The drawing under review shows one solid part. Ordinate dimensions are in mm from its lowest x, y, z. A direction names the side the tool comes from. Coordinates: 2 decimals unless noted, no trailing zeros. Order: outer loops, then holes, each group sorted by start corner. A loop starts at its lowest first (then second) coordinate and runs counter-clockwise, first axis right, second up. Notation, with made-up numbers: (51.5, 24) -> (107.5, 24) arc R22 cw to (107.5, 56) -> close; hole circle Ø8 at (88, -28.75). An arc over 180 degrees is marked (long way). Put each result on its own line as item: value.
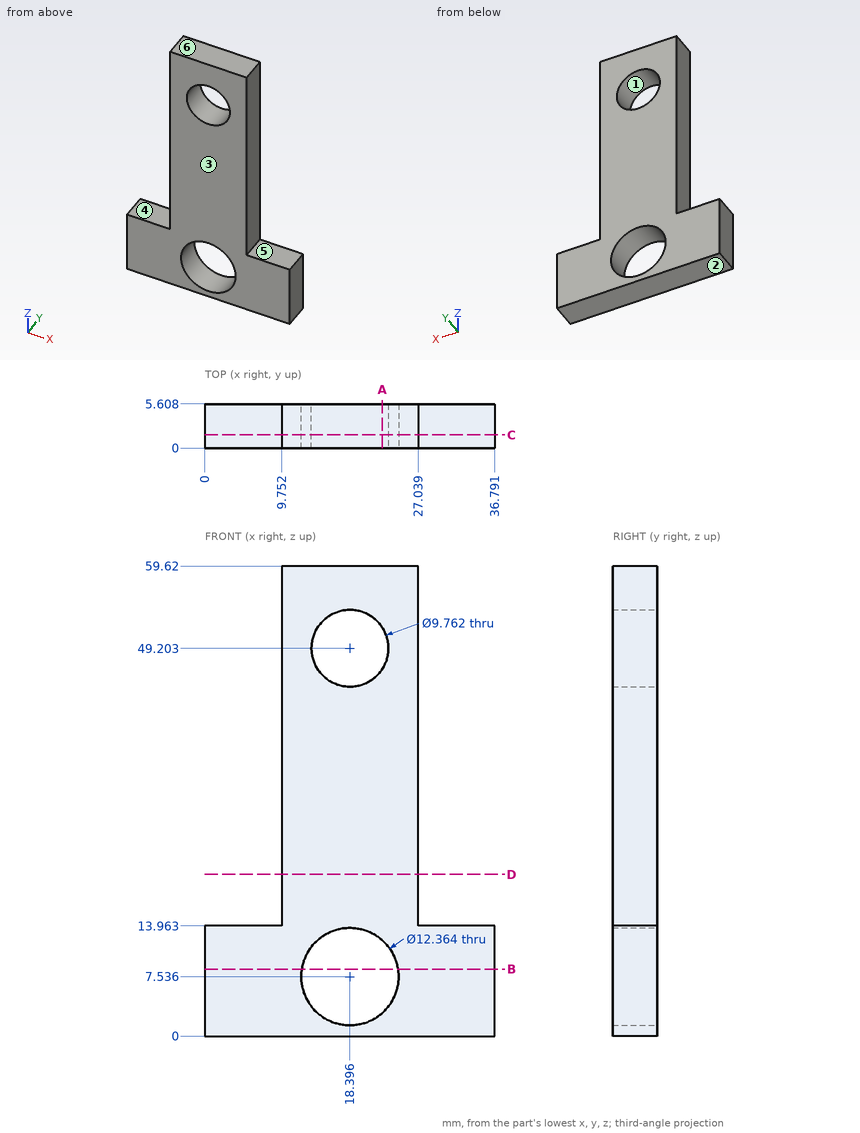
Item 1: Consider section D-D on z = 20.5. Write out the cut boundary in (x, y).
Answers below:
outline: (9.75, 0) -> (27.04, 0) -> (27.04, 5.61) -> (9.75, 5.61) -> close
Item 2: For line 1 (Z direction, x = 33, y = 2.75); line 2 (X direction, y = 2.3, z = 14.5); line 3 (Z direction, x = 24, y = 1.6) (1 decimal), list the stretches that pass through material, from the lowest coordinate up. Write a range as from..to.
Answers below:
line 1: 0..13.96
line 2: 9.75..27.04
line 3: 0..4.9, 10.1..59.6
Item 3: Consider section C-C on y = 1.7. Write out the cut boundary in (x, z) (1 decimal), and give its area (3 significant figures).
Answers below:
outline: (0, 0) -> (36.8, 0) -> (36.8, 14) -> (27, 14) -> (27, 59.6) -> (9.8, 59.6) -> (9.8, 14) -> (0, 14) -> close; hole circle Ø12.4 at (18.4, 7.5); hole circle Ø9.8 at (18.4, 49.2)
area: 1,110 mm^2
Item 4: For the marked faces 5 and 6, list the 3-axis set-ups (+Z, -Z, +X, -X, +Y, -Y) from which the entire face can be reached by the end or side of a thin tool; tool diameter is ignored.
Answers below:
face 5: +Z, +X, +Y, -Y
face 6: +Z, +X, -X, +Y, -Y
Item 5: Consider section A-A on x = 22.5. Write out the cut boundary in (y, z) (1 decimal), and give its area (3 significant figures).
Answers below:
outline: (0, 0) -> (5.6, 0) -> (5.6, 2.9) -> (0, 2.9) -> close; (0, 12.2) -> (5.6, 12.2) -> (5.6, 46.6) -> (0, 46.6) -> close; (0, 51.8) -> (5.6, 51.8) -> (5.6, 59.6) -> (0, 59.6) -> close
area: 253 mm^2
Item 6: Consider section B-B on z = 8.5. Write out the cut boundary in (x, y), and give its area (3 significant figures).
Answers below:
outline: (0, 0) -> (12.29, 0) -> (12.29, 5.61) -> (0, 5.61) -> close; (24.5, 0) -> (36.79, 0) -> (36.79, 5.61) -> (24.5, 5.61) -> close
area: 138 mm^2
Item 7: Mouldability with a two-part tool opening along Z and no side actions: class the marked faces 1, 2, 3 and 4 as +Z half, -Z half, draft (parallel to the pull), parting line (faces both ways), or undercut.
Answers below:
face 1: undercut
face 2: -Z half
face 3: draft
face 4: +Z half
Item 8: For pin 1 Ø12.5 at (x, z) = (18.4, 49.2) entering from +Y; pin 2 Ø1.7 at (x, y) = (3, 3.5) entering from +Z; pin 3 Ø3 at (y, z) = (4, 38) entering from -X, all flat-tipped, find the tip position at first contact; note any pin that passes through.
Answers below:
pin 1: y = 5.61
pin 2: z = 13.96
pin 3: x = 9.75
